The listing builds one solid part. Answer for the finished solid, in the listing's coordinates (mm). Face numbers are marked on the shaded views. Coordinates: 2 decimals unless noted, no trailing zeros. Order: outer loops, then holes, each group sorted by start corner. A loop starts at its lowest first (then second) coordinate and runs counter-clockwise, first axis right, second up.
```python
from build123d import *

# Parameters (mm, degrees)
SKETCH1_W           = 700
SKETCH1_H           = 200
BOSS_EXTRUDE1_DEPTH = 650
CUT_EXTRUDE2_DEPTH  = 680
SKETCH7_W           = 650
SKETCH7_H           = 200
BOSS_EXTRUDE3_DEPTH = 20


with BuildPart() as part:
    # Sketch1 → Boss-Extrude1 (new body)
    with BuildSketch(Plane.XY):
        Rectangle(SKETCH1_W, SKETCH1_H)
    extrude(amount=-BOSS_EXTRUDE1_DEPTH)

    # Sketch6 → Cut-Extrude2 (cut)
    with BuildSketch(Plane(origin=(350, 0, 0), x_dir=(0, 0, -1), z_dir=(1, 0, 0))):
        with BuildLine():
            Line((0, 85), (0, -85))
            ThreePointArc((0, -85), (330.583898703, -50.56807643), (626.895433751, 100))
            Line((626.895433751, 100), (16.346883748, 100))
            ThreePointArc((16.346883748, 100), (11.280043592, 89.114449525), (0, 85))
        make_face()
    extrude(amount=-CUT_EXTRUDE2_DEPTH, mode=Mode.SUBTRACT)

    # Sketch7 → Boss-Extrude3 (add)
    with BuildSketch(Plane(origin=(350, 0, 0), x_dir=(0, 0, -1), z_dir=(1, 0, 0))):
        with Locations((325, 0)):
            Rectangle(SKETCH7_W, SKETCH7_H)
    extrude(amount=BOSS_EXTRUDE3_DEPTH)


solid = part.part
```
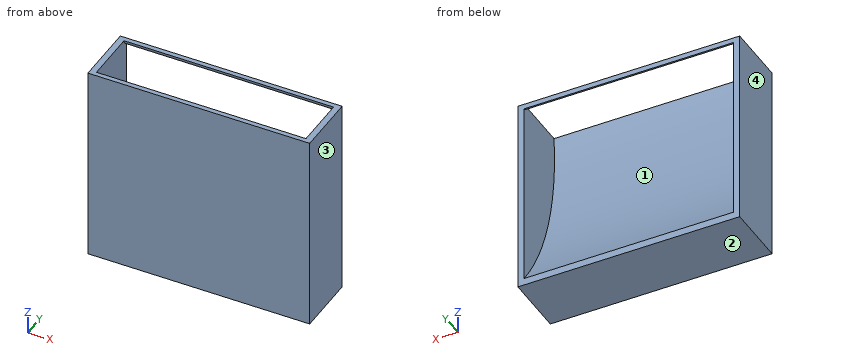
1) Straight lines are drawn through the part: probe 1 along X at (y, z) = (43.5, -314.5); probe 2 along Y at (x, z) = (187.5, -90); probe 3 along Y at (x, z) = (-240.5, -340). For each, find the intervals that lie inside material, in ascending order.
2) A cutting plane is placed at A-A, the plane x = 27.5. Write down the section's boundary in (y, z), plus the area to 3 significant figures.
3) The mould has two halves that part along X. Classify the marked faces 1, 2, 3 and 4: released by +X, released by -X, zero draft, split by the parting line, or undercut.
4) A cutting plane is placed at B-B, the plane z = -106.5. Write down the section's boundary in (x, y), plus the area to 3 significant figures.
5) Each of these flat-tipped pins is pushed along its axis until it touches: P1, Ø12, axis at x = 221.5, y = -16, coming from the +Z side; P2, Ø8, axis at x = -224, z = -462.5, coming from the +Y side. Where does it stop, or does it pass through?
6) A cutting plane is placed at C-C, the plane y = -18.5. Write down the section's boundary in (x, z), plus the area to 3 significant figures.
Working result:
1. probe 1: x = -350 to -330, 350 to 370
1. probe 2: y = -100 to -87.7
1. probe 3: y = -100 to -47.73
2. outline: (-100, -650) - (100, -650) - (100, -626.9) arc R912.33 cw to (-85, 0) - (-100, 0) - close; (85, 0) arc R15.69 ccw to (100, -16.35) - (100, 0) - close
2. area: 45,600 mm2
3. face 1: undercut
3. face 2: zero draft
3. face 3: released by +X
3. face 4: released by -X
4. outline: (-350, -100) - (370, -100) - (370, 100) - (350, 100) - (350, -87.24) - (-330, -87.24) - (-330, 100) - (-350, 100) - close
4. area: 16,700 mm2
5. P1: stops at z = -412.74
5. P2: stops at y = 1.66
6. outline: (-350, -650) - (370, -650) - (370, 0) - (350, 0) - (350, -421.32) - (-330, -421.32) - (-330, 0) - (-350, 0) - close
6. area: 182,000 mm2
